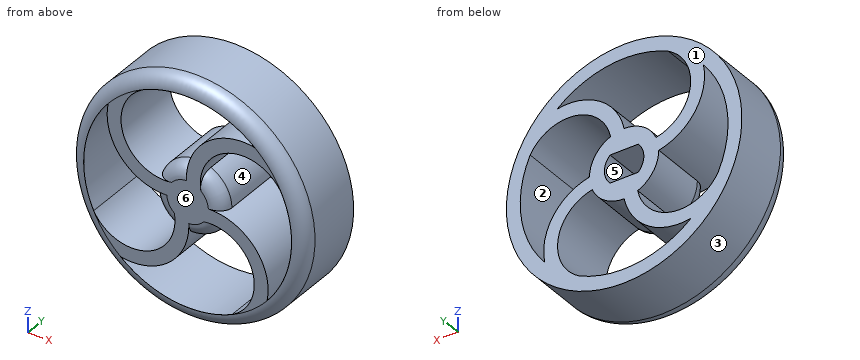
```python
from build123d import *

# Parameters (mm, degrees)
SKETCH1_R           = 17
SKETCH1_R_2         = 14.999999999999998
BOSS_EXTRUDE1_DEPTH = 10
SKETCH2_R           = 5
BOSS_EXTRUDE2_DEPTH = 10
BOSS_EXTRUDE3_START = -10
BOSS_EXTRUDE3_DEPTH = 10
FILLET1_R           = 2
BOSS_EXTRUDE4_START = -2
BOSS_EXTRUDE4_DEPTH = 2
FILLET2_R           = 2
CUT_EXTRUDE1_DEPTH  = 8


with BuildPart() as part:
    # Sketch1 → Boss-Extrude1 (new body)
    with BuildSketch(Plane(origin=(0, 0, 0), x_dir=(1, 0, 0), z_dir=(0, 1, 0))):
        with Locations(Location((0, 0, 0), (0, 0, 270))):
            Circle(SKETCH1_R)
        with Locations(Location((0, 0, 0), (0, 0, 270))):
            Circle(SKETCH1_R_2, mode=Mode.SUBTRACT)
    extrude(amount=BOSS_EXTRUDE1_DEPTH)



with BuildPart() as body_2:
    # Sketch2 → Boss-Extrude2 (new body)
    with BuildSketch(Plane(origin=(0, 10, 0), x_dir=(1, 0, 0), z_dir=(0, 1, 0))):
        with Locations(Location((0, 0, 0), (0, 0, 270))):
            Circle(SKETCH2_R)
        with BuildLine():
            Line((-1.9448650338776723, 1.8000000000000003), (1.9448650338776723, 1.8000000000000003))
            ThreePointArc((1.9448650338776723, 1.8000000000000003), (2.65, 2.9e-16), (1.9448650338776725, -1.8))
            Line((1.9448650338776725, -1.8), (-1.9448650338776725, -1.8))
            ThreePointArc((-1.9448650338776725, -1.8), (-2.65, 3.2e-16), (-1.9448650338776723, 1.8000000000000003))
        make_face(mode=Mode.SUBTRACT)
    extrude(amount=-BOSS_EXTRUDE2_DEPTH)


with BuildPart() as part_1:
    add(part.part)

    add(body_2.part)  # Boss-Extrude3 merges body 2
    # Sketch3 → Boss-Extrude3 (add)
    with BuildSketch(Plane(origin=(0, 10, 0), x_dir=(1, 0, 0), z_dir=(0, 1, 0)).offset(BOSS_EXTRUDE3_START)):
        with BuildLine():
            ThreePointArc((-13.566134305689296, 6.4), (-7.136792678521299, 9.536951322914675), (-1.9595917942265426, 4.6000000000000005))
            ThreePointArc((-1.9595917942265426, 4.6000000000000005), (-1.0000000000000004, 4.898979485566357), (0, 5.000000000000001))
            ThreePointArc((0, 5.000000000000001), (-3.511067317848477, 10.221869444049297), (-9.681023203858528, 11.457652016288186))
            ThreePointArc((-9.681023203858528, 11.457652016288186), (-11.895484187198832, 9.137694236080705), (-13.566134305689296, 6.4))
        make_face()
        with BuildLine():
            ThreePointArc((6.400000000000048, 13.566134305689273), (9.5369513229147, 7.1367926785212665), (4.600000000000008, 1.9595917942265266))
            ThreePointArc((4.600000000000008, 1.9595917942265266), (4.898979485566361, 0.9999999999999829), (5.000000000000001, -1.746e-14))
            ThreePointArc((5.000000000000001, -1.746e-14), (10.221869444049313, 3.5110673178484406), (11.45765201628822, 9.681023203858487))
            ThreePointArc((11.45765201628822, 9.681023203858487), (9.137694236080746, 11.895484187198797), (6.400000000000048, 13.566134305689273))
        make_face()
        with BuildLine():
            ThreePointArc((13.56613430568925, -6.4000000000000945), (7.136792678521233, -9.536951322914723), (1.9595917942265106, -4.600000000000015))
            ThreePointArc((1.9595917942265106, -4.600000000000015), (0.9999999999999661, -4.898979485566364), (-3.491e-14, -5.000000000000001))
            ThreePointArc((-3.491e-14, -5.000000000000001), (3.511067317848407, -10.221869444049325), (9.681023203858448, -11.457652016288254))
            ThreePointArc((9.681023203858448, -11.457652016288254), (11.895484187198766, -9.137694236080788), (13.56613430568925, -6.4000000000000945))
        make_face()
        with BuildLine():
            ThreePointArc((-6.4000000000001425, -13.566134305689229), (-9.53695132291475, -7.1367926785212), (-4.600000000000022, -1.9595917942264942))
            ThreePointArc((-4.600000000000022, -1.9595917942264942), (-4.898979485566368, -0.9999999999999478), (-5.000000000000001, 5.281e-14))
            ThreePointArc((-5.000000000000001, 5.281e-14), (-10.221869444049336, -3.5110673178483705), (-11.457652016288288, -9.681023203858407))
            ThreePointArc((-11.457652016288288, -9.681023203858407), (-9.13769423608083, -11.895484187198734), (-6.4000000000001425, -13.566134305689229))
        make_face()
    extrude(amount=BOSS_EXTRUDE3_DEPTH)

    # Fillet1
    fillet1_edges = [part_1.edges().sort_by_distance(p)[0] for p in [
        (5.2e-15, 0, -17),
    ]]
    fillet(fillet1_edges, radius=FILLET1_R - 0.0001)  # a hair under: the kernel refuses the full size

    # Sketch4 → Boss-Extrude4 (add)
    with BuildSketch(Plane.XZ.offset(BOSS_EXTRUDE4_START)):
        with BuildLine():
            Line((-1.9448650338776725, 1.8), (1.9448650338776725, 1.8))
            ThreePointArc((1.9448650338776725, 1.8), (2.65, 0), (1.9448650338776723, -1.8000000000000003))
            Line((1.9448650338776723, -1.8000000000000003), (-1.9448650338776723, -1.8000000000000003))
            ThreePointArc((-1.9448650338776723, -1.8000000000000003), (-2.65, 3.2e-16), (-1.9448650338776725, 1.8))
        make_face()
    extrude(amount=BOSS_EXTRUDE4_DEPTH)

    # Fillet2
    fillet2_edges = [part_1.edges().sort_by_distance(p)[0] for p in [
        (-4.171208396324286, 0, -2.7569948339512305),
        (2.7569948339512154, 0, -4.171208396324297),
        (4.171208396324286, 0, 2.7569948339512305),
        (-2.7569948339512305, 0, 4.171208396324286),
    ]]
    fillet(fillet2_edges, radius=FILLET2_R)

    # Sketch5 → Cut-Extrude1 (cut)
    with BuildSketch(Plane(origin=(0, 10, 0), x_dir=(1, 0, 0), z_dir=(0, 1, 0))):
        with BuildLine():
            Line((-2.030394050424718, -2), (2.0303940504247175, -2.0000000000000004))
            ThreePointArc((2.0303940504247175, -2.0000000000000004), (2.850000000000016, -3.2e-16), (2.030394050424718, 2))
            Line((2.030394050424718, 2), (-2.030394050424718, 2))
            ThreePointArc((-2.030394050424718, 2), (-2.850000000000016, 3.5e-16), (-2.030394050424718, -2))
        make_face()
    extrude(amount=-CUT_EXTRUDE1_DEPTH, mode=Mode.SUBTRACT)


solid = part_1.part
```
The model under review builds one solid part; all positions refer to its coordinate system, in mm. Face numbers are marked on the shaded views. A direction names the side the tool comes from. Round coordinates to 2 decimals unless told otherwise and drop trailing zeros. Loops run counter-clockwise (first coordinate to the right, second up) from the corner with the lowest first, then second, coordinate; pieces in that order, holes last. Notation, with made-up numbers: M 68.25,-5 L 105.25,-5 A15 ccw 105.25,12 Z; hole C 83.25,27.5 d2. An arc over 180 degrees is marked long. Put each result on its own line as item: value.
Q1. Machinability: for the marked faces 4, 5 and 6, which of the approach directions +Z, -Z, +X, -X, +Y, -Y give a long, thin tool a straight path to every point of the face, cutting with its end or side? Answer none if there is none.
Result set:
face 4: +Y, -Y
face 5: +Y
face 6: +Z, -Z, +X, -X, -Y
Q2. Consider section A-A, the plane y = 6. Give the boundary of the cut face in (x, z), then the cut area to 3 significant figures.
Result set:
outline: C 0,0 d34; hole M -13.57,-6.4 A6.26 ccw -1.96,-4.6 A5 cw -5,0 A8.26 cw -11.46,9.68 A15 ccw Z; hole M -9.68,-11.46 A15 ccw 6.4,-13.57 A6.26 ccw 4.6,-1.96 A5 cw 0,-5 A8.26 cw Z; hole M -6.4,13.57 A6.26 ccw -4.6,1.96 A5 cw 0,5 A8.26 cw 9.68,11.46 A15 ccw Z; hole M -2.03,-2 L 2.03,-2 A2.85 ccw 2.03,2 L -2.03,2 A2.85 ccw Z; hole M 1.96,4.6 A5 cw 5,0 A8.26 cw 11.46,-9.68 A15 ccw 13.57,6.4 A6.26 ccw Z
area: 366 mm²
Q3. For pin 1 (3 mm diameter, centred on x = 2.5, y = 2.5, fed in from +Z); pin 2 (3 mm diameter, centred on x = -5.5, y = 1, fed in from -Z); pin 3 (1.2 mm diameter, centred on x = -1, z = 1, fed in from +Y), all flat-tipped, find the tip position at first contact; note any pin that passes through.
Result set:
pin 1: stops at z = 16.97
pin 2: stops at z = -16.46
pin 3: stops at y = 2
Q4. Consider section B-B, the plane z = 7. Count the separate pieces of the cut face and the enclosed holes in it, then the cut area to 3 significant figures.
Result set:
separate pieces: 4
enclosed holes: 0
area: 86.9 mm²
Q5. To check wall thickness, follow L1, parallel to X at y = 9.5, z = 1.5; L2, parallel to Z at x = 6.5, y = 5.5; L3, parallel to Z at x = 5.5, y = 1.75. State the ranges of each line that lie inside material, in increasing order.
Result set:
L1: x = -16.93 to -14.92, -8.32 to -2.42, 2.42 to 4.77, 14.92 to 16.93
L2: z = -15.71 to -13.51, -2.68 to -0.46, 9.4 to 11.46, 13.52 to 15.71
L3: z = -16.07 to -13.96, -2.21 to -0.12, 9.05 to 11.19, 13.96 to 16.07
Q6. Mouldability with a two-part tool opening along X and no side actions: class the marked faces 1, 2 and 3 as released by +X, released by -X, zero draft, split by the parting line, or undercut.
Result set:
face 1: zero draft
face 2: undercut
face 3: split by the parting line
